from build123d import *

# Parameters (mm, degrees)
SKETCH3_R           = 3.302
BOSS_EXTRUDE2_DEPTH = 6.35
CUT_EXTRUDE3_DEPTH  = 450.865121453
FILLET2_R           = 6.35
FILLET3_R           = 2.54
FILLET4_R           = 2.54
FILLET5_R           = 6.35
FILLET6_R           = 2.54
FILLET7_R           = 2.54


with BuildPart() as part:
    # Sketch3 → Boss-Extrude2 (new body)
    with BuildSketch(Plane(origin=(0, 0, 0), x_dir=(-1, 0, 0), z_dir=(0, 1, 0))):
        with BuildLine():
            Line((48.352684633, -96.934831966), (326.488935594, -297.252717824))
            ThreePointArc((326.488935594, -297.252717824), (333.094584687, -297.751891673), (336.55, -292.1))
            Line((336.55, -292.1), (336.55, -152.4))
            ThreePointArc((336.55, -152.4), (335.66916846, -149.173438927), (333.271040518, -146.842013841))
            Line((333.271040518, -146.842013841), (166.415977763, -54.646991456))
            ThreePointArc((166.415977763, -54.646991456), (164.068228098, -53.896304985), (161.611498988, -54.096156795))
            Line((161.611498988, -54.096156795), (50.330310781, -85.673293323))
            ThreePointArc((50.330310781, -85.673293323), (45.809453277, -90.683804291), (48.352684633, -96.934831966))
        make_face()
        with Locations(Location((52.063749039, -91.782114142, 0), (0, 0, 90))):
            Circle(SKETCH3_R, mode=Mode.SUBTRACT)
        with Locations(Location((163.344937246, -60.204977615, 0), (0, 0, 90))):
            Circle(SKETCH3_R, mode=Mode.SUBTRACT)
        with Locations(Location((330.2, -152.4, 0), (0, 0, 90))):
            Circle(SKETCH3_R, mode=Mode.SUBTRACT)
        with Locations(Location((330.2, -292.1, 0), (0, 0, 90))):
            Circle(SKETCH3_R, mode=Mode.SUBTRACT)
    extrude(amount=BOSS_EXTRUDE2_DEPTH)

    # Sketch9 → Cut-Extrude3 (cut, through all)
    with BuildSketch(Plane(origin=(0, 6.35, 0), x_dir=(1, 0, 0), z_dir=(0, 1, 0))):
        Polygon((-326.39, 284.660691911), (-201.3623279, 194.613893401), (-326.39, 159.064940036), align=None)
        Polygon((-319.046617377, 150.590173625), (-195.643102449, 185.677332519), (-170.986081265, 68.779983296), align=None)
        Polygon((-184.597750493, 182.539794136), (-60.685190052, 93.296115712), (-159.839017865, 65.160237505), align=None)
    extrude(amount=-CUT_EXTRUDE3_DEPTH, mode=Mode.SUBTRACT)

    # Fillet2
    fillet2_edges = [part.edges().sort_by_distance(p)[0] for p in [
        (-159.839017865, 3.175, -65.160237505),
    ]]
    fillet(fillet2_edges, radius=FILLET2_R)

    # Fillet3
    fillet3_edges = [part.edges().sort_by_distance(p)[0] for p in [
        (-170.986081265, 3.175, -68.779983296),
    ]]
    fillet(fillet3_edges, radius=FILLET3_R)

    # Fillet4
    fillet4_edges = [part.edges().sort_by_distance(p)[0] for p in [
        (-319.046617377, 3.175, -150.590173625),
    ]]
    fillet(fillet4_edges, radius=FILLET4_R)

    # Fillet5
    fillet5_edges = [part.edges().sort_by_distance(p)[0] for p in [
        (-326.39, 3.175, -159.064940036),
    ]]
    fillet(fillet5_edges, radius=FILLET5_R)

    # Fillet6
    fillet6_edges = [part.edges().sort_by_distance(p)[0] for p in [
        (-60.685190052, 3.175, -93.296115712),
        (-326.39, 3.175, -284.660691911),
    ]]
    fillet(fillet6_edges, radius=FILLET6_R)

    # Fillet7
    fillet7_edges = [part.edges().sort_by_distance(p)[0] for p in [
        (-195.643102449, 3.175, -185.677332519),
        (-184.597750493, 3.175, -182.539794136),
        (-201.3623279, 3.175, -194.613893401),
    ]]
    fillet(fillet7_edges, radius=FILLET7_R)


solid = part.part
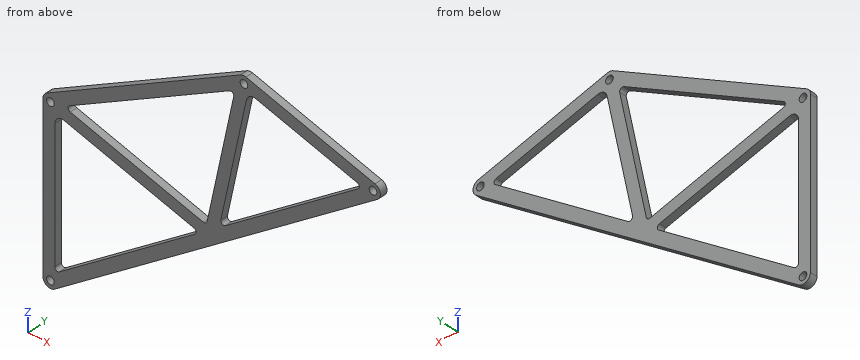
Could you check a few things on this model? Use its own coordinates, in mm. Round coordinates to 2 decimals unless told otherwise and drop trailing zeros. Loops run counter-clockwise (first coordinate to the right, second up) from the corner with the lowest first, then second, coordinate; pieces in that order, holes last. Notation, with made-up numbers: (37, 86.25) -> (42, 86.25) arc R17 cw to (42, 90.25) -> close; hole circle Ø3 at (-3.75, -10.75). An arc over 180 degrees is marked (long way). Use CSV: the item, a comma, the result in double quotes.
(1) Will these pins go through, and if not, where does the flat tip stop? pin 1 Ø6 at (x, z) = (-330.2, -292.1) entering from -Y; pin 2 Ø1.5 at (x, y) = (-224, 5) entering from +Z; pin 3 Ø1.9 at (y, z) = (4, -251) entering from +X.
Return value:
pin 1,"passes through"
pin 2,"stops at z = -86.05"
pin 3,"stops at x = -260.95"
(2) If I drill on probe 1 along X at (y, z) = (2, -110.5); probe 2 along Z at (x, y) = (-238, 5.5); probe 3 along Z at (x, y) = (-283, 5), over which ranges is the centre line in solid material (lowest first)? Write a range as [from, to].
Return value:
probe 1,"x = [-267.5, -246.49], [-179.79, -169.4], [-84.57, -67.19]"
probe 2,"z = [-233.52, -221], [-184.2, -173.63], [-105.81, -94.2]"
probe 3,"z = [-265.93, -253.41], [-171.4, -160.84], [-130.67, -119.06]"
(3) Suppose I cut it at B-B on z = -260.5. Write out the boundary of the cut face in (x, y), plus the area to 3 significant figures.
Return value:
outline,"(-336.55, 0) -> (-326.39, 0) -> (-326.39, 6.35) -> (-336.55, 6.35) -> close; (-292.84, 0) -> (-275.46, 0) -> (-275.46, 6.35) -> (-292.84, 6.35) -> close"
area,"175 mm²"
(4) Suppose I cut it at A-A on y = 4.5. Give the number of separate pieces and of enclosed holes in the cut face, plus the area to 3 significant figures.
Return value:
separate pieces,"1"
enclosed holes,"7"
area,"10,600 mm²"
(5) Suppose I cut it at C-C on x = -288.5. Write out the boundary of the cut face in (y, z).
Return value:
outline,"(0, -269.89) -> (6.35, -269.89) -> (6.35, -257.37) -> (0, -257.37) -> close; (0, -169.84) -> (6.35, -169.84) -> (6.35, -159.28) -> (0, -159.28) -> close; (0, -133.71) -> (6.35, -133.71) -> (6.35, -122.1) -> (0, -122.1) -> close"
(6) Suppose I cut it at D-D on z = -116.5. Write out the boundary of the cut face in (x, y), plus the area to 3 significant figures.
Return value:
outline,"(-278.36, 0) -> (-257.35, 0) -> (-257.35, 6.35) -> (-278.36, 6.35) -> close; (-181.05, 0) -> (-170.67, 0) -> (-170.67, 6.35) -> (-181.05, 6.35) -> close; (-92.9, 0) -> (-75.52, 0) -> (-75.52, 6.35) -> (-92.9, 6.35) -> close"
area,"310 mm²"
